from build123d import *

# Parameters (mm, degrees)
PADR_OCIRCULAR1_COUNT = 4
FILETE1_R             = 0.5


with BuildPart() as part:
    # Esboço1 → Revolução1 (revolve)
    with BuildSketch(Plane(origin=(0, 0, 0), x_dir=(0, 0, -1), z_dir=(1, 0, 0)), mode=Mode.PRIVATE) as revolu_o1_sk:
        Polygon((0, 25), (0, 32.25), (-0.5, 32.25), (-0.5, 32.75), (0, 32.75), (0, 39.5), (-0.5, 39.5), (-0.5, 40), (0, 40), (0, 58), (-13, 58), (-13, 40), (-100, 40), (-100, 32.75), (-99.5, 32.75), (-99.5, 32.25), (-100, 32.25), (-100, 25), align=None)
    revolve(revolu_o1_sk.sketch.rotate(Axis((0, 0, 0), (0, 0, 1)), 90), axis=Axis((0, 0, 0), (0, 0, 1)))  # turned: the seam where the file's is

    # Esboço5 → Corte-Revolução1 (revolve, cut)
    with BuildSketch(Plane(origin=(0, 0, 0), x_dir=(0, 0, -1), z_dir=(1, 0, 0)), mode=Mode.PRIVATE) as corte_revolu_o1_sk:
        Polygon((0, 56), (-8.1, 56), (-8.1, 53.5), (-13, 53.5), (-13, 49), (0, 49), align=None)
    corte_revolu_o1 = revolve(corte_revolu_o1_sk.sketch.rotate(Axis((0, 49, 0), (0, 0, -1)), 90), axis=Axis((0, 49, 0), (0, 0, -1)), mode=Mode.SUBTRACT)  # turned: the seam where the file's is

    # PadrãoCircular1: Corte-Revolução1 ×4 about axis
    padr_ocircular1_axis = Axis((0, 0, 0), (0, 0, 1))
    for i in range(1, PADR_OCIRCULAR1_COUNT):
        add(corte_revolu_o1.rotate(padr_ocircular1_axis, i * 360 / PADR_OCIRCULAR1_COUNT), mode=Mode.SUBTRACT)

    # Filete1
    filete1_edges = [part.edges().sort_by_distance(p)[0] for p in [
        (40, 0, 100),
        (58, 0, 13),
        (58, 0, 0),
    ]]
    fillet(filete1_edges, radius=FILETE1_R)


solid = part.part
Here's how the part is built. I have some questions about the finished solid (model axes, mm). A direction names the side the tool comes from. Give positions to 0.01 mm unless a question says otherwise; leave off trailing zeros. Loops run counter-clockwise (first coordinate to the right, second up) from the corner with the lowest first, then second, coordinate; pieces in that order, holes last. Notation, with made-up numbers: (-35.5, -11.5) -> (-22.5, -11.5) arc R15 cw to (-22.5, -7.5) -> close; hole circle Ø5 at (-25, 16). An arc over 180 degrees is marked (long way). One line per item, written item: value.
Q1. Suppose I cut it at B-B on x = 0. State how many separate pieces and enclosed holes the cut face has, then the cut area to 3 significant figures.
Answers follow:
separate pieces: 4
enclosed holes: 0
area: 3,150 mm^2
Q2. I'm going to push flat-ended pins straight in: pin 1 Ø1.5 at (x, z) = (-37, 18.5) entering from -Y; pin 2 Ø11 at (x, y) = (-49, 0.5) entering from -Z; pin 3 Ø3 at (x, z) = (-7.5, 39.5) entering from +Y; pin 4 Ø8 at (x, y) = (0, 49) entering from +Z. Where does each tip first touch, or does it pass through?
Answers follow:
pin 1: y = -16.91
pin 2: z = 8.1
pin 3: y = 39.55
pin 4: through
Q3. If I drill on line 1 along Y through (x, z) = (0, 10.5); line 2 along Y through (x, z) = (0, 4.25); line 3 along Z through (x, y) = (10, 52), over which ranges is the centre line in solid material (lowest first)?
Answers follow:
line 1: -58 to -53.5, -44.5 to -25, 25 to 44.5, 53.5 to 58
line 2: -58 to -56, -42 to -25, 25 to 42, 56 to 58
line 3: 0 to 13
Q4. We'd pull the mould along X, two halves only. Please class faces 1 (the face through (-31.238, -9.837, 0.246)), 2 (the face through (53.39, 0.98, 10.58)), 3 (the face through (39.96, -1.76, 56.86)), 4 (the face through (-34.3, 21, 0)): pulls with the +X half, pulls with the -X half, needs draft (parallel to the pull), parting line crosses it, or undercut.
Answers follow:
face 1: undercut
face 2: undercut
face 3: parting line crosses it
face 4: needs draft
Q5. On a 3-axis mill with a long thin cutter (end or side, diameter ignored), from which of +Z, -Z, +X, -X, +Y, -Y can I reach the whole of each face in a straight line? I mean faces 5 (the face through (-31.238, -9.837, 99.746)), 6 (the face through (-53.39, -0.98, 10.58)), 7 (the face through (0.91, -42.06, 4.11)). Say none if no direction works.
Answers follow:
face 5: +Z
face 6: +Z, -Z
face 7: -Z
Q6. Suppose I cut it at A-A on z = 38. Please give me the cut outline in (x, y).
Answers follow:
outline: circle Ø80 at (0, 0); hole circle Ø50 at (0, 0)
